Autodesk Inventor part; units mm, degrees
ref_plane "YZ Plane" through (0, 0, 0) normal (1, 0, 0) x (0, 1, 0)
ref_plane "XZ Plane" through (0, 0, 0) normal (0, 1, 0) x (-1, 0, 0)
ref_plane "XY Plane" through (0, 0, 0) normal (0, 0, 1) x (1, 0, 0)
sketch "Sketch1" plane through (0, 0, 0) normal (0, 1, 0) x (-1, 0, 0)
  circle A0 centre (0, 0) radius 50.8
  circle A1 centre (0, 0) radius 20.32
  dimension "d0" = 101.6
  dimension "d1" = 40.64
extrude "Extrusion1" add sketch "Sketch1" along normal blind 10.16
sketch "Sketch2" plane through (0, 10.16, 0) normal (0, 1, 0) x (1, 0, 0)
  circle A0 centre (0, 0) radius 47.625
  dimension "d4" = 95.25
extrude "Extrusion2" cut sketch "Sketch2" against normal blind 6.35
sketch "Sketch3" plane through (0, 10.16, 0) normal (0, 1, 0) x (1, 0, 0)
  circle A0 centre (0, 0) radius 47.625
  line L0 (-47.625, 0) -> (-57.785, 0)
  line L1 (-57.785, 0) -> (-57.785, 10.16)
  line L2 (-57.785, 10.16) -> (-47.625, 10.16)
  line L3 (-47.625, 10.16) -> (-47.625, -10.16)
  line L4 (-47.625, -10.16) -> (-57.785, -10.16)
  line L5 (-57.785, -10.16) -> (-57.785, 0)
  line L6 (0, 47.625) -> (0, 57.785)
  line L7 (0, 57.785) -> (10.16, 57.785)
  line L8 (10.16, 57.785) -> (10.16, 47.625)
  line L9 (10.16, 47.625) -> (-10.16, 47.625)
  line L10 (-10.16, 47.625) -> (-10.16, 57.785)
  line L11 (-10.16, 57.785) -> (0, 57.785)
  line L12 (47.625, 0) -> (57.785, 0)
  line L13 (57.785, 0) -> (57.785, 10.16)
  line L14 (57.785, 10.16) -> (47.625, 10.16)
  line L15 (47.625, 10.16) -> (47.625, -10.16)
  line L16 (47.625, -10.16) -> (57.785, -10.16)
  line L17 (57.785, -10.16) -> (57.785, 0)
  line L18 (0, -47.625) -> (0, -57.785)
  line L19 (0, -57.785) -> (10.16, -57.785)
  line L20 (10.16, -57.785) -> (10.16, -47.625)
  line L21 (10.16, -47.625) -> (-10.16, -47.625)
  line L22 (-10.16, -47.625) -> (-10.16, -57.785)
  line L23 (-10.16, -57.785) -> (0, -57.785)
  dimension "d7" = 10.16
  dimension "d8" = 10.16
  dimension "d9" = 20.32
  dimension "d10" = 10.16
  dimension "d11" = 10.16
  dimension "d12" = 10.16
  dimension "d13" = 20.32
  dimension "d14" = 10.16
  dimension "d15" = 10.16
  dimension "d16" = 10.16
  dimension "d17" = 20.32
  dimension "d18" = 10.16
  dimension "d19" = 10.16
  dimension "d20" = 10.16
  dimension "d21" = 10.16
  dimension "d22" = 20.32
  dimension "d23" = 10.16
extrude "Extrusion3" add sketch "Sketch3" against normal up to surface (10.16 mm away) contours L21 L20 L19 L18 | L18 L23 L22 L21 | L3 L4 L5 L0 | L0 L1 L2 L3 | L9 L10 L11 L6 | L6 L7 L8 L9 | L15 L14 L13 L12 | L12 L17 L16 L15
sketch "Sketch4" plane through (0, 10.16, 0) normal (0, 1, 0) x (1, 0, 0)
  line L0 (-57.785, 10.16) -> (-57.785, -10.16)
  line L1 (-57.785, 10.16) -> (-52.705, 10.16)
  line L2 (-49.7736, 10.16) -> (-57.785, 10.16)
  line L3 (-52.705, 10.16) -> (-52.705, 5.08)
  line L4 (-52.705, 5.08) -> (-52.705, -5.08)
  line L5 (-10.16, 57.785) -> (-10.16, 49.7736)
  line L6 (-10.16, 57.785) -> (-10.16, 52.705)
  line L7 (-10.16, 52.705) -> (-5.08, 52.705)
  line L8 (-5.08, 52.705) -> (5.08, 52.705)
  line L9 (49.7736, 10.16) -> (57.785, 10.16)
  line L10 (57.785, 10.16) -> (52.705, 10.16)
  line L11 (52.705, 10.16) -> (52.705, 5.08)
  line L12 (52.705, 5.08) -> (52.705, -5.08)
  line L13 (10.16, -49.7736) -> (10.16, -57.785)
  line L14 (10.16, -57.785) -> (10.16, -52.705)
  line L15 (10.16, -52.705) -> (5.08, -52.705)
  line L16 (5.08, -52.705) -> (-5.08, -52.705)
  circle A0 centre (-52.705, -5.08) radius 2.2479
  circle A1 centre (-52.705, 5.08) radius 2.2479
  circle A2 centre (-5.08, 52.705) radius 2.2479
  circle A3 centre (5.08, 52.705) radius 2.2479
  circle A4 centre (52.705, 5.08) radius 2.2479
  circle A5 centre (52.705, -5.08) radius 2.2479
  circle A6 centre (-5.08, -52.705) radius 2.2479
  circle A7 centre (5.08, -52.705) radius 2.2479
  point P0 (0, 0)
  dimension "d26" = 5.08
  dimension "d27" = 5.08
  dimension "d28" = 10.16
  dimension "d29" = 5.08
  dimension "d30" = 5.08
  dimension "d31" = 10.16
  dimension "d32" = 5.08
  dimension "d33" = 5.08
  dimension "d34" = 10.16
  dimension "d35" = 5.08
  dimension "d36" = 5.08
  dimension "d37" = 10.16
  dimension "d38" = 4.4958
  dimension "d39" = 4.4958
  dimension "d40" = 4.4958
  dimension "d41" = 4.4958
  dimension "d42" = 4.4958
  dimension "d43" = 4.4958
  dimension "d44" = 4.4958
extrude "Extrusion4" cut sketch "Sketch4" against normal blind 25.4
properties part number "CO-0-01-PlanetaryCap"
Read the model definition and answer for the solid it produces. Units are mm, in the model's axes. A direction names the side the tool comes from. Coordinates: 2 decimals unless noted, no trailing zeros. Write each loop counter-clockwise with the first axis right and the second up, starting at its lowest first coordinate (ties: lowest second). Pieces come first, ordered by that corner, then holes. Notation, with made-up numbers: (5, 72) - (18, 72) arc R21 ccw to (18, 80) - close; hole circle Ø3 at (71, 79). An arc over 180 degrees is marked (long way). Answer as a JSON object with one key per item and string values. Group by question number.
1. A cutting plane is placed at D-D (z = 39.5). Determine the outline of the cut face in (x, y).
2. A cutting plane is placed at B-B (z = 0). Determine the outline of the cut face in (x, y) (3 decimals).
3. A cutting plane is placed at A-A (x = 0). Determine the outline of the cut face in (y, z) (3 decimals), plus the area to 3 significant figures.
4. Consider L1, parallel to Z at x = 0, y = 7.25 (3 decimals); L2, parallel to Z at x = -4.5, y = 1.25 (3 decimals); L3, parallel to X at y = 2.2, z = 0 (3 decimals). Determine where each line is inside the solid, lowest interval first. Write a range as [from, to].
5. The mould has two halves that part along Z. Classify faces 5 (the cylindrical face through (-36.21, 5.01, -35.63)), 6 (the cylindrical face through (-35.63, 5.01, 36.21)), 7 (the flat face through (-10.16, 5, -54)), 8 (the cylindrical face through (4.787, 5.151, -54.934)): +Z half, -Z half, draft (parallel to the pull), parting line (faces both ways), or undercut.
6. Which of the six approach directions +Z, -Z, +X, -X, +Y, -Y give full straight-line access (tool end or side, diameter ignored) to faces 1 (the flat face through (54, 5, 10.16)), 2 (the flat face through (-54, 5, -10.16)), 3 (the flat face through (-10.16, 5, 54)), 4 (the flat face through (10.16, 5, -54))?
7. Each of these flat-tipped pins is pushed along its axis until it touches: P1, Ø5, axis at y = 2, z = 27, coming from the -X side; P2, Ø4, axis at x = -55.5, y = 3.5, coming from the +Z side; P3, Ø3, axis at y = 3, z = -41, coming from the -X side. Where does it stop, or does it pass through?
8. A cutting plane is placed at C-C (y = 8.25). Give the number of separate pieces and of enclosed holes in the cut face, plus the area to 3 significant figures.
Worked out:
{
 "1": {"outline": "(-31.94, 0) - (31.94, 0) - (31.94, 10.16) - (26.61, 10.16) - (26.61, 3.81) - (-26.61, 3.81) - (-26.61, 10.16) - (-31.94, 10.16) - close"},
 "2": {"outline": "(-57.785, 0) - (-20.32, 0) - (-20.32, 3.81) - (-47.625, 3.81) - (-47.625, 10.16) - (-57.785, 10.16) - close; (20.32, 0) - (57.785, 0) - (57.785, 10.16) - (47.625, 10.16) - (47.625, 3.81) - (20.32, 3.81) - close"},
 "3": {"outline": "(0, -57.785) - (10.16, -57.785) - (10.16, -47.625) - (3.81, -47.625) - (3.81, -20.32) - (0, -20.32) - close; (0, 20.32) - (3.81, 20.32) - (3.81, 47.625) - (10.16, 47.625) - (10.16, 57.785) - (0, 57.785) - close", "area": "415 mm²"},
 "4": {"L1": "z = [-57.785, -47.625], [47.625, 57.785]", "L2": "z = [-57.785, -54.877], [-50.533, -19.815], [19.815, 50.533], [54.877, 57.785]", "L3": "x = [-57.785, -20.32], [20.32, 57.785]"},
 "5": {"face 5": "-Z half", "face 6": "+Z half", "face 7": "draft", "face 8": "undercut"},
 "6": {"face 1": "+Z, +X, +Y, -Y", "face 2": "-Z, -X, +Y, -Y", "face 3": "+Z, -X, +Y, -Y", "face 4": "-Z, +X, +Y, -Y"},
 "7": {"P1": "stops at x = -44.5", "P2": "stops at z = 10.16", "P3": "stops at x = -31.94"},
 "8": {"separate pieces": "1", "enclosed holes": "9", "area": "1,450 mm²"}
}
